Check sheet for the modelled part. Datum: model origin and axes. Units: mm. A direction names the side the tool comes from. Coordinates: 2 decimals unless noted, no trailing zeros. Loops run counter-clockwise (first coordinate to the right, second up) from the corner with the lowest first, then second, coordinate; pieces in that order, holes last. Notation, with made-up numbers: (-18, 15) -> (38, 15) arc R20 cw to (38, 51) -> close; hole circle Ø10 at (8, 58.5). An arc over 180 degrees is marked (long way). Use CSV: the item, a comma, the result in double quotes.
```python
from build123d import *

# Parameters (mm, degrees)
PAD004_DEPTH = 3
PAD_DEPTH    = 6
PAD002_DEPTH = 6
PAD003_DEPTH = 3
PAD001_DEPTH = 6


with BuildPart() as counterborehole_pad:
    # Sketch004 → Pad004 (new body)
    with BuildSketch(Plane.XY.offset(3)):
        with BuildLine():
            ThreePointArc((-15, -93.000008), (-11.999996, -96), (-9, -93))
            Line((-9, -90), (-9, -93))
            ThreePointArc((-9, -90), (-12, -87), (-15, -90.000001))
            Line((-15, -90.000001), (-15, -93.000008))
        make_face()
        with BuildLine():
            ThreePointArc((15, -90.000001), (12, -87), (9, -90))
            Line((9, -90), (9, -93))
            ThreePointArc((9, -93), (11.999996, -96), (15, -93.000008))
            Line((15, -90.000001), (15, -93.000008))
        make_face()
    extrude(amount=PAD004_DEPTH)


with BuildPart() as throughhole_pad:
    # Sketch003 → Pad (new body)
    with BuildSketch(Plane.XY):
        with BuildLine():
            ThreePointArc((-10.25, -90), (-12.000001, -88.25), (-13.75, -90.000003))
            Line((-13.75, -90.000003), (-13.75, -93))
            ThreePointArc((-13.75, -93), (-12, -94.75), (-10.25, -93))
            Line((-10.25, -90), (-10.25, -93))
        make_face()
        with BuildLine():
            ThreePointArc((13.75, -90.000003), (12.000001, -88.25), (10.25, -90))
            Line((10.25, -90), (10.25, -93))
            ThreePointArc((10.25, -93), (12, -94.75), (13.75, -93))
            Line((13.75, -90.000003), (13.75, -93))
        make_face()
    extrude(amount=PAD_DEPTH)


with BuildPart() as frame_pad:
    # Sketch002 → Pad002 (new body)
    with BuildSketch(Plane.XY):
        with BuildLine():
            ThreePointArc((-30, -79.529869), (0, -85), (30, -79.529869))
            Line((30, -79.529869), (30, -85.912746))
            ThreePointArc((-30, -85.912746), (0, -91), (30, -85.912746))
            Line((-30, -85.912746), (-30, -79.529869))
        make_face()
    extrude(amount=PAD002_DEPTH)


with BuildPart() as base_pad:
    # Sketch001 → Pad003 (new body)
    with BuildSketch(Plane.XY):
        with BuildLine():
            ThreePointArc((8.560325, -69.83078), (0, -65), (-8.560325, -69.83078))
            Line((-20, -88.774996), (-8.560325, -69.83078))
            ThreePointArc((-20, -88.774996), (0, -91), (20, -88.774996))
            Line((8.560325, -69.83078), (20, -88.774996))
        make_face()
    extrude(amount=PAD003_DEPTH)


with BuildPart() as counterborehole_cut:
    # Sketch → Pad001 (new body)
    with BuildSketch(Plane.XY):
        with BuildLine():
            ThreePointArc((-20, -82.613558), (0, -85), (20, -82.613558))
            Line((20, -82.613558), (20, -99.299958))
            Line((20, -99.299958), (-20, -99.299958))
            Line((-20, -99.299958), (-20, -82.613558))
        make_face()
    extrude(amount=PAD001_DEPTH)

    # Fusion: union Frame_Pad, Base_Pad
    add(frame_pad.part)
    add(base_pad.part)

    # Cut: cut ThroughHole_Pad
    add(throughhole_pad.part, mode=Mode.SUBTRACT)

    # Cut001: cut CounterboreHole_Pad
    add(counterborehole_pad.part, mode=Mode.SUBTRACT)


solid = counterborehole_cut.part
```
1) Access from +Z, -Z, +X, -X, +Y, -Y to the whole of each face (thin tool, end or side, straight path). Record for faces 4 (the flat face through (-20, -94, 3)), 5 (the flat face through (-15, -91, 4)), 6 (the cylindrical face through (-11.96, -88.25, 1.48)).
Answer below:
face 4,"+Z, -Z, -X, -Y"
face 5,"+Z"
face 6,"+Z, -Z"
2) Cross-section at B-B on z = 1.3. Record the boundary of the cut face in (x, y) (3 decimals).
Answer below:
outline,"(-30, -85.913) arc R91 ccw to (-20, -88.775) -> (-20, -99.3) -> (20, -99.3) -> (20, -88.775) arc R91 ccw to (30, -85.913) -> (30, -79.53) arc R85 cw to (20, -82.614) arc R85 cw to (16.718, -83.34) -> (8.56, -69.831) arc R10 ccw to (-8.56, -69.831) -> (-16.718, -83.34) arc R85 cw to (-20, -82.614) arc R85 cw to (-30, -79.53) -> close; hole (-13.75, -93) arc R1.75 ccw to (-10.25, -93) -> (-10.25, -90) arc R1.75 ccw to (-13.75, -90) -> close; hole (10.25, -93) arc R1.75 ccw to (13.75, -93) -> (13.75, -90) arc R1.75 ccw to (10.25, -90) -> close"
3) Thickness scan on line 1 along X through (y, z) = (-91.5, 4.6); line 2 along X through (y, z) = (-91, 2.5); line 3 along Z through (x, y) = (-7, -72.5). Record the ranges inside material, lowest first. Write a range as from..to.
Answer below:
line 1,"x = -20..-15, -9..9, 15..20"
line 2,"x = -20..-13.75, -10.25..10.25, 13.75..20"
line 3,"z = 0..3"
4) Cross-section at C-C on z = 3.9. Record the boundary of the cut face in (x, y) (3 decimals).
Answer below:
outline,"(-30, -85.913) arc R91 ccw to (-20, -88.775) -> (-20, -99.3) -> (20, -99.3) -> (20, -88.775) arc R91 ccw to (30, -85.913) -> (30, -79.53) arc R85 cw to (20, -82.614) arc R85 cw to (-20, -82.614) arc R85 cw to (-30, -79.53) -> close; hole (-15, -93) arc R3 ccw to (-9, -93) -> (-9, -90) arc R3 ccw to (-15, -90) -> close; hole (9, -93) arc R3 ccw to (15, -93) -> (15, -90) arc R3 ccw to (9, -90) -> close"
5) Cross-section at D-D on x = -18. Record the boundary of the cut face in (y, z), and give its area (3 significant figures).
Answer below:
outline,"(-99.3, 0) -> (-83.07, 0) -> (-83.07, 6) -> (-99.3, 6) -> close"
area,"97.4 mm²"
6) Cross-section at A-A on x = 12. Record the boundary of the cut face in (y, z).
Answer below:
outline,"(-99.3, 0) -> (-94.75, 0) -> (-94.75, 3) -> (-96, 3) -> (-96, 6) -> (-99.3, 6) -> close; (-88.25, 0) -> (-75.53, 0) -> (-75.53, 3) -> (-84.15, 3) -> (-84.15, 6) -> (-87, 6) -> (-87, 3) -> (-88.25, 3) -> close"
7) Go/stop test with flat-tipped pins: pin 1 Ø1 at (y, z) = (-93.5, 2) entering from -X; pin 2 Ø16 at (x, y) = (2.5, -74.5) entering from +Z; pin 3 Ø1.5 at (x, z) = (17.5, 5) entering from +Y. Record where each tip stops, or that it passes through.
Answer below:
pin 1,"stops at x = -20"
pin 2,"stops at z = 3"
pin 3,"stops at y = -83.02"
8) Draft check along Y on faces 1 (the flat face through (13.75, -91, 1)), 2 (the cylindrical face through (0, -65, 1)), 3 (the flat face through (-30, -83, 3)). Enter one of: released by +Y, released by -Y, zero draft, split by the parting line, or undercut.
Answer below:
face 1,"undercut"
face 2,"released by +Y"
face 3,"zero draft"
